Check sheet for the modelled part. Datum: model origin and axes. Units: mm. Face numbers are marked on the shaded views. A direction names the side the tool comes from. Give positions to 0.01 mm unless a question says otherwise; leave off trailing zeros. Loops run counter-clockwise (first coordinate to the right, second up) from the corner with the lowest first, then second, coordinate; pieces in that order, holes last.
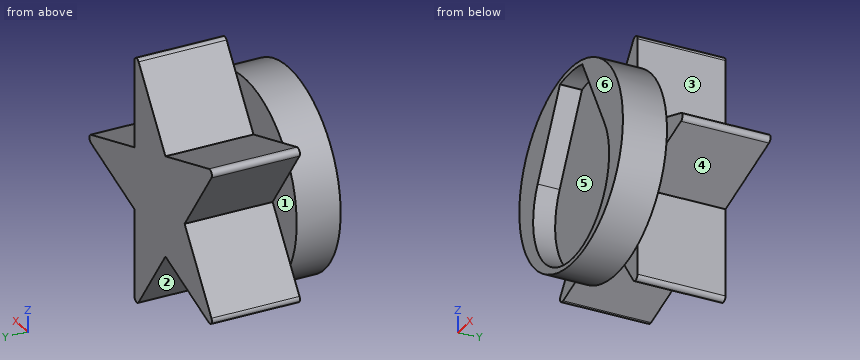
```python
from build123d import *

# Parameters (mm, degrees)
SKETCH1_R           = 22.5
BOSS_EXTRUDE1_DEPTH = 10
BOSS_EXTRUDE2_DEPTH = 20
SKETCH3_R           = 16.5
CUT_EXTRUDE2_DEPTH  = 5


with BuildPart() as part:
    # Sketch1 → Boss-Extrude1 (new body)
    with BuildSketch(Plane(origin=(0, 0, 0), x_dir=(1, 0, 0), z_dir=(0, 1, 0))):
        Circle(SKETCH1_R)
    extrude(amount=BOSS_EXTRUDE1_DEPTH)

    # Sketch2 → Boss-Extrude2 (add)
    with BuildSketch(Plane(origin=(0, 10, 0), x_dir=(1, 0, 0), z_dir=(0, 1, 0))):
        with BuildLine():
            Line((9.747590887, 26.922316463), (9.747590887, 7.082039325))
            Line((9.747590887, 7.082039325), (28.616815744, 0.951056516))
            ThreePointArc((28.616815744, 0.951056516), (29.30779875, 0), (28.616815744, -0.951056516))
            Line((28.616815744, -0.951056516), (9.747590887, -7.082039325))
            Line((9.747590887, -7.082039325), (9.747590887, -26.922316463))
            ThreePointArc((9.747590887, -26.922316463), (9.056607881, -27.873372979), (7.938573893, -27.510101715))
            Line((7.938573893, -27.510101715), (-3.72324841, -11.458980338))
            Line((-3.72324841, -11.458980338), (-22.592473267, -17.589963146))
            ThreePointArc((-22.592473267, -17.589963146), (-23.710507256, -17.226691882), (-23.710507256, -16.051121378))
            Line((-23.710507256, -16.051121378), (-12.048684953, 0))
            Line((-12.048684953, 0), (-23.710507256, 16.051121378))
            ThreePointArc((-23.710507256, 16.051121378), (-23.710507256, 17.226691882), (-22.592473267, 17.589963146))
            Line((-22.592473267, 17.589963146), (-3.72324841, 11.458980338))
            Line((-3.72324841, 11.458980338), (7.938573893, 27.510101715))
            ThreePointArc((7.938573893, 27.510101715), (9.056607881, 27.873372979), (9.747590887, 26.922316463))
        make_face()
    extrude(amount=BOSS_EXTRUDE2_DEPTH)

    # Sketch3 → Cut-Extrude2 (cut)
    with BuildSketch(Plane.XZ):
        with BuildLine():
            ThreePointArc((-14.551420086, 2.778571429), (0, 11.5), (14.551420086, 2.778571429))
            Line((14.551420086, 2.778571429), (4.83856504, 20.948467447))
            ThreePointArc((4.83856504, 20.948467447), (0, 21.5), (-4.83856504, 20.948467447))
            Line((-4.83856504, 20.948467447), (-14.551420086, 2.778571429))
        make_face()
        with Locations((0, -5)):
            Circle(SKETCH3_R)
    extrude(amount=-CUT_EXTRUDE2_DEPTH, mode=Mode.SUBTRACT)


solid = part.part
```
(1) Gauge pin test, flat ends, axial feed: pin 1 Ø1.5 at (y, z) = (26.5, 1) entering from +X; pin 2 Ø1 at (x, y) = (-13.5, 4) entering from +Z; pin 3 Ø12 at (x, z) = (6.5, -6.5) entering from -Y. Record the tip position at first contact, or that the pin passes through.
(2) Section check B-B on x = 0. Record the boundary of the cut face in (y, z), plus the area to 3 significant figures.
(3) Release check for a two-part mould opening along X. For the marked faces 4, 5 and 6 record: pulls with the +X half, pulls with the -X half, needs draft (parallel to the pull), parting line crosses it, or undercut.
(4) Material ranges on line 1 (Y direction, x = -3.5, z = 16.5); line 2 (Y direction, x = -7, z = 8.5); line 3 (X direction, y = 1.6, z = -5), recorded low to high.
(5) Access from +Z, -Z, +X, -X, +Y, -Y to the whole of each face (thin tool, end or side, straight path). Record for the marked faces 1, 2 and 3.
(6) Section check A-A on y = 26.5. Record the boundary of the cut face in (x, z).
(7) Section check D-D on y = 3.5. Record the boundary of the cut face in (x, z).
(8) Section check C-C on z = -5. Record the boundary of the cut face in (x, y).
Computed values:
1. pin 1: stops at x = 29.28
1. pin 2: stops at z = 18.36
1. pin 3: stops at y = 5
2. outline: (0, -22.5) - (10, -22.5) - (10, -16.58) - (30, -16.58) - (30, 16.58) - (10, 16.58) - (10, 22.5) - (0, 22.5) - (0, 21.5) - (5, 21.5) - (5, -21.5) - (0, -21.5) - close
2. area: 898 mm2
3. face 4: pulls with the +X half
3. face 5: undercut
3. face 6: needs draft
4. line 1: y = 5 to 10
4. line 2: y = 5 to 30
4. line 3: x = -21.94 to -16.5, 16.5 to 21.94
5. face 1: -X, +Y
5. face 2: -Z, +Y
5. face 3: +Z, +X, +Y
6. outline: (-23.71, -16.05) arc R1 ccw to (-22.59, -17.59) - (-3.72, -11.46) - (7.94, -27.51) arc R1 ccw to (9.75, -26.92) - (9.75, -7.08) - (28.62, -0.95) arc R1 ccw to (28.62, 0.95) - (9.75, 7.08) - (9.75, 26.92) arc R1 ccw to (7.94, 27.51) - (-3.72, 11.46) - (-22.59, 17.59) arc R1 ccw to (-23.71, 16.05) - (-12.05, 0) - close
7. outline: circle Ø45 at (0, 0); hole (-14.55, 2.78) arc R16.5 ccw (long way) to (14.55, 2.78) - (4.84, 20.95) arc R21.5 ccw to (-4.84, 20.95) - close
8. outline: (-21.94, 0) - (-16.5, 0) - (-16.5, 5) - (16.5, 5) - (16.5, 0) - (21.94, 0) - (21.94, 10) - (16.16, 10) - (16.16, 30) - (-15.68, 30) - (-15.68, 10) - (-21.94, 10) - close
